The model under review builds one solid part; all positions refer to its coordinate system, in mm. Face numbers are marked on the shaded views. Coordinates: 2 decimals unless noted, no trailing zeros. Order: outer loops, then holes, each group sorted by start corner. A loop starts at its lowest first (then second) coordinate and runs counter-clockwise, first axis right, second up. Notation, with made-up numbers: (-37, 6.5) -> (16, 6.5) arc R9 cw to (16, 17.5) -> close; hole circle Ø7 at (-38.5, -9). An arc over 180 degrees is marked (long way). Use one line per item in the form item = value.
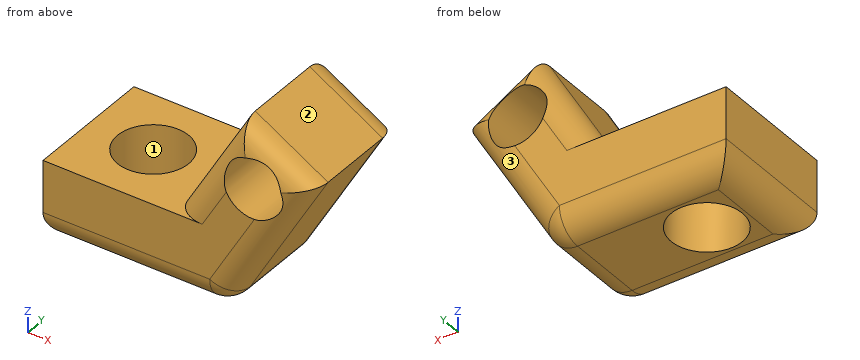
from build123d import *

# Parameters (mm, degrees)
EXTRUDE_1_DEPTH          = 10
CUT_EXTRUDE_1_DEPTH      = 29.347234569
CUT_EXTRUDE_1_DEPTH_BACK = 29.347234569
SKETCH_2_R               = 2.75
SKETCH_3_R               = 2.25
CUT_EXTRUDE_2_DEPTH      = 27.669152308
FILLET_1_R               = 2


with BuildPart() as part:
    # Эскиз1 → Бобышка-Вытянуть1 (new body)
    with BuildSketch(Plane(origin=(0, 0, 0), x_dir=(1, 0, 0), z_dir=(0, 1, 0))):
        Polygon((-22.105263158, 3.587719298), (-22.105263158, -2.412280702), (-12.105263158, -2.412280702), (-7.105263158, -11.07253474), (-1.476098033, -7.82253474), (-8.063811274, 3.587719298), align=None)
    extrude(amount=EXTRUDE_1_DEPTH)

    # Эскиз2 → Вырез-Вытянуть1 (cut, two sides: drawn at the far end of the back side and taken through both)
    with BuildSketch(Plane(origin=(0, 0, -3.587719298), x_dir=(-1, 0, 0), z_dir=(0, 0, -1)).offset(-CUT_EXTRUDE_1_DEPTH_BACK)):
        with Locations((17.105263158, 5)):
            Circle(SKETCH_2_R)
    extrude(amount=CUT_EXTRUDE_1_DEPTH + CUT_EXTRUDE_1_DEPTH_BACK, mode=Mode.SUBTRACT)

    # Эскиз3 → Вырез-Вытянуть2 (cut, through all)
    with BuildSketch(Plane.XZ):
        with Locations(Location((-5.915680596, 6.632952177, 0), (0, 0, 270))):
            Circle(SKETCH_3_R)
    extrude(amount=-CUT_EXTRUDE_2_DEPTH, mode=Mode.SUBTRACT)

    # Скругление1
    # the kernel refuses this fillet: 2 mm, written as the material it takes off along each edge
    with BuildSketch(Plane(origin=(-9.218511812, 2, -1.587719298), x_dir=(0.8660254037844398, 0, -0.499999999999998), z_dir=(0, -1, 0))) as fillet_1_piece_1_section:
        Polygon((0, 0), (FILLET_1_R, 0), (FILLET_1_R, -FILLET_1_R * 0.57735026919), (FILLET_1_R * 0.5, -FILLET_1_R * 0.866025403784), align=None)
    fillet_1_piece_1 = extrude(amount=FILLET_1_R, mode=Mode.PRIVATE)
    fillet_1_piece_1 = fillet_1_piece_1 - Plane(origin=(-9.218511812, 2, -1.587719298), x_dir=(-0.500000000000001, 0, 0.8660254037844382), z_dir=(0, -1, 0)) * Sphere(FILLET_1_R, mode=Mode.PRIVATE)
    add(fillet_1_piece_1, mode=Mode.SUBTRACT)
    with BuildSketch(Plane(origin=(-9.218511812, 8, -1.587719298), x_dir=(0.8660254037844398, 0, -0.499999999999998), z_dir=(0, 1, 0))) as fillet_1_piece_2_section:
        Polygon((0, 0), (FILLET_1_R, 0), (FILLET_1_R, FILLET_1_R * 0.57735026919), (FILLET_1_R * 0.5, FILLET_1_R * 0.866025403784), align=None)
    fillet_1_piece_2 = extrude(amount=FILLET_1_R, mode=Mode.PRIVATE)
    fillet_1_piece_2 = fillet_1_piece_2 - Plane(origin=(-9.218511812, 8, -1.587719298), x_dir=(-0.500000000000001, 0, 0.8660254037844382), z_dir=(0, 1, 0)) * Sphere(FILLET_1_R, mode=Mode.PRIVATE)
    add(fillet_1_piece_2, mode=Mode.SUBTRACT)
    with BuildSketch(Plane(origin=(-8.063811274, 2, -3.587719298), x_dir=(-1, 0, 0), z_dir=(0, 1, 0))) as fillet_1_piece_3:
        with BuildLine():
            CenterArc((FILLET_1_R * 0.57735026919, FILLET_1_R), FILLET_1_R, 210, 60)
            Line((-FILLET_1_R * 0.288675134595, FILLET_1_R * 0.5), (0, 0))
            Line((0, 0), (FILLET_1_R * 0.57735026919, 0))
        make_face()
    extrude(amount=6, mode=Mode.SUBTRACT)
    with BuildSketch(Plane(origin=(-22.105263158, -5, -3.587719298), x_dir=(0, 0, 1), z_dir=(0, 1, 0))) as fillet_1_piece_4:
        with BuildLine():
            CenterArc((FILLET_1_R, FILLET_1_R), FILLET_1_R, 180, 90)
            Line((0, FILLET_1_R), (0, 0))
            Line((0, 0), (FILLET_1_R, 0))
        make_face()
    extrude(amount=20, mode=Mode.SUBTRACT)
    with BuildSketch(Plane(origin=(-14.605263158, 10, -1.917846317), x_dir=(0.8660254037844399, 0, -0.4999999999999979), z_dir=(0.49999999999999795, 0, 0.8660254037844399))) as fillet_1_piece_5_section:
        with BuildLine():
            CenterArc((FILLET_1_R, -FILLET_1_R), FILLET_1_R, 90, 90)
            Line((0, -FILLET_1_R), (0, 0))
            Line((0, 0), (FILLET_1_R, 0))
        make_face()
    fillet_1_piece_5 = extrude(amount=20, mode=Mode.PRIVATE)
    fillet_1_piece_5 = split(fillet_1_piece_5, bisect_by=Plane(origin=(-7.90513861, 9.542907556, 2.412280702), z_dir=(0, 0, 1)), keep=Keep.TOP, mode=Mode.PRIVATE)
    add(fillet_1_piece_5, mode=Mode.SUBTRACT)
    with BuildSketch(Plane(origin=(-11.435390177, 10, 13.57253474), x_dir=(-0.4999999999999979, 0, -0.8660254037844399), z_dir=(0.8660254037844399, 0, -0.49999999999999795))) as fillet_1_piece_6:
        with BuildLine():
            CenterArc((FILLET_1_R, -FILLET_1_R), FILLET_1_R, 90, 90)
            Line((0, -FILLET_1_R), (0, 0))
            Line((0, 0), (FILLET_1_R, 0))
        make_face()
    extrude(amount=16.5, mode=Mode.SUBTRACT)
    with BuildSketch(Plane(origin=(1.023901967, 10, 12.152661759), x_dir=(-0.8660254037844398, 0, 0.499999999999998), z_dir=(-0.499999999999998, 0, -0.8660254037844398))) as fillet_1_piece_7:
        with BuildLine():
            CenterArc((FILLET_1_R, -FILLET_1_R), FILLET_1_R, 90, 90)
            Line((0, -FILLET_1_R), (0, 0))
            Line((0, 0), (FILLET_1_R, 0))
        make_face()
    extrude(amount=17.020725942, mode=Mode.SUBTRACT)
    with BuildSketch(Plane(origin=(-9.218511812, 10, -3.587719298), x_dir=(0, -1, 0), z_dir=(-1, 0, 0))) as fillet_1_piece_8:
        with BuildLine():
            CenterArc((FILLET_1_R, FILLET_1_R), FILLET_1_R, 180, 90)
            Line((0, FILLET_1_R), (0, 0))
            Line((0, 0), (FILLET_1_R, 0))
        make_face()
    extrude(amount=17.886751346, mode=Mode.SUBTRACT)
    with BuildSketch(Plane(origin=(1.023901967, 0, 12.152661759), x_dir=(-0.8660254037844398, 0, 0.499999999999998), z_dir=(-0.499999999999998, 0, -0.8660254037844398))) as fillet_1_piece_9:
        with BuildLine():
            CenterArc((FILLET_1_R, FILLET_1_R), FILLET_1_R, 180, 90)
            Line((0, FILLET_1_R), (0, 0))
            Line((0, 0), (FILLET_1_R, 0))
        make_face()
    extrude(amount=17.020725942, mode=Mode.SUBTRACT)
    with BuildSketch(Plane(origin=(-11.435390177, 0, 13.57253474), x_dir=(-0.4999999999999979, 0, -0.8660254037844399), z_dir=(0.8660254037844399, 0, -0.49999999999999795))) as fillet_1_piece_10:
        with BuildLine():
            CenterArc((FILLET_1_R, FILLET_1_R), FILLET_1_R, 180, 90)
            Line((0, FILLET_1_R), (0, 0))
            Line((0, 0), (FILLET_1_R, 0))
        make_face()
    extrude(amount=16.5, mode=Mode.SUBTRACT)
    with BuildSketch(Plane(origin=(-14.605263158, 0, -1.917846317), x_dir=(0.8660254037844398, 0, -0.4999999999999979), z_dir=(0.49999999999999795, 0, 0.8660254037844399))) as fillet_1_piece_11_section:
        with BuildLine():
            CenterArc((FILLET_1_R, FILLET_1_R), FILLET_1_R, 180, 90)
            Line((0, FILLET_1_R), (0, 0))
            Line((0, 0), (FILLET_1_R, 0))
        make_face()
    fillet_1_piece_11 = extrude(amount=20, mode=Mode.PRIVATE)
    fillet_1_piece_11 = split(fillet_1_piece_11, bisect_by=Plane(origin=(-7.90513861, 0.457092444, 2.412280702), z_dir=(0, 0, 1)), keep=Keep.TOP, mode=Mode.PRIVATE)
    add(fillet_1_piece_11, mode=Mode.SUBTRACT)
    with BuildSketch(Plane(origin=(-9.218511812, 0, -3.587719298), x_dir=(0, 1, 0), z_dir=(-1, 0, 0))) as fillet_1_piece_12:
        with BuildLine():
            CenterArc((FILLET_1_R, -FILLET_1_R), FILLET_1_R, 90, 90)
            Line((0, -FILLET_1_R), (0, 0))
            Line((0, 0), (FILLET_1_R, 0))
        make_face()
    extrude(amount=17.886751346, mode=Mode.SUBTRACT)


solid = part.part
Item 1: Draft analysis for pull direction Y (two halves, no side actions). For the marked faces 1, 2 and 3, state which applies: released by +Y, released by -Y, zero draft, split by the parting line, or undercut.
Results found:
face_1 = undercut
face_2 = zero draft
face_3 = released by +Y
Item 2: We need section B-B (x = -18.75). Write out the cut boundary in (y, z).
Results found:
outline = (0, -1.59) arc R2 ccw to (2, -3.59) -> (2.8, -3.59) -> (2.8, 2.41) -> (0, 2.41) -> close; (7.2, -3.59) -> (8, -3.59) arc R2 ccw to (10, -1.59) -> (10, 2.41) -> (7.2, 2.41) -> close
Item 3: Clearance check with flat-ended pins moving along their axes: pin 1 (4 mm diameter, centred on x = -19, y = 5, fed in from -Z); pin 2 (4 mm diameter, centred on x = -5.92, z = 6.63, fed in from +Y); pin 3 (4 mm diameter, centred on x = -4.5, y = 6, fed in from +Z). State where each tip first meets the part, or that it passes through.
Results found:
pin_1 = -3.59
pin_2 = through
pin_3 = 10.72
Item 4: We need section A-A (y = 5). Write out the cut boundary in (x, z).
Results found:
outline = (-22.11, -1.59) arc R2 ccw to (-20.11, -3.59) -> (-19.86, -3.59) -> (-19.86, 2.41) -> (-22.11, 2.41) -> close; (-14.36, -3.59) -> (-9.22, -3.59) arc R2 ccw to (-7.49, -2.59) -> (-1.48, 7.82) -> (-7.11, 11.07) -> (-12.11, 2.41) -> (-14.36, 2.41) -> close; hole circle Ø4.5 at (-5.92, 6.63)
Item 5: To check wall thickness, follow L1, parallel to Z at x = -14, y = 3; L2, parallel to X at y = 3.25, z = -2.5; L3, parallel to Z at x = -7.5, y = 2. State the ranges of each line that lie inside material, in increasing order. Write a range as from..to.
Results found:
L1 = -3.59..2.41
L2 = -21.89..-19.23, -14.98..-7.44
L3 = -2.61..5.04, 8.23..10.39
Item 6: We need section C-C (y = 6.75). Write out the cut boundary in (x, z).
Results found:
outline = (-22.11, -1.59) arc R2 ccw to (-20.11, -3.59) -> (-19.23, -3.59) -> (-19.23, 2.41) -> (-22.11, 2.41) -> close; (-14.98, -3.59) -> (-9.22, -3.59) arc R2 ccw to (-7.49, -2.59) -> (-1.48, 7.82) -> (-7.11, 11.07) -> (-12.11, 2.41) -> (-14.98, 2.41) -> close; hole circle Ø4.5 at (-5.92, 6.63)
